CAD build for the part. Positions are in the model's coordinates, mm. Face numbers are marked on the shaded views. A direction names the side the tool comes from. Give positions to 0.01 mm unless a question says otherwise; leave off trailing zeros. Write each loop counter-clockwise with the first axis right and the second up, starting at its lowest first coordinate (ties: lowest second). Pieces come first, ordered by that corner, then holes. Notation, with made-up numbers: (21.5, 28.5) - (79.5, 28.5) arc R29 cw to (79.5, 66.5) - close; hole circle Ø8 at (-21, 41). An arc over 180 degrees is marked (long way). Put each result on its own line as item: value. Start each with the question number.
1. Drop flat-ended pins along their axis: pin 1 (1.5 mm diameter, centred on y = 454.5, z = 22, fed in from -X); pin 2 (11.5 mm diameter, centred on x = 22.5, z = 0, fed in from -Y); pin 3 (4 mm diameter, centred on y = 219.5, z = 0.5, fed in from +X); pin 4 (1 mm diameter, centred on x = 13, y = 62, fed in from -Z). Give the stop position or say it passes through.
2. Wall check: line 1 (Z direction, x = 0, y = 450.05); line 2 (X direction, y = 455.1, z = 0); line 3 (Z direction, x = 22.5, y = 451.1). Give the ranges that are in metal, low to high.
3. Tool access for the marked faces 4, 5 and 6: list every direction of +Z, -Z, +X, -X, +Y, -Y with a clear straight run to the whole face (end or side of a thin tool).
4. Mould opens along Y. For the marked faces 1, 2 and 3 say: +Y half, -Y half, draft (parallel to the pull), parting line (faces both ways), or undercut.
5. Cut at A-A on y = 79. List the corners of the cut face in (x, z), and give its area (3 significant figures).
from build123d import *

# Parameters (mm, degrees)
SKETCH1_W                     = 30
SKETCH1_H                     = 30
BOSS_EXTRUDE1_DEPTH           = 458
SKETCH2_W                     = 15
SKETCH2_H                     = 30
SKETCH2_W_2                   = 30
SKETCH2_H_2                   = 15
BOSS_EXTRUDE2_DEPTH           = 10
CBORE_FOR_M5_SHCS1_AT_2_COUNT = 2
CBORE_FOR_M5_SHCS1_AT_2_PITCH = 45
CBORE_FOR_M5_SHCS1_AT_3_COUNT = 2
CBORE_FOR_M5_SHCS1_AT_3_PITCH = 31.819805153
CBORE_FOR_M5_SHCS1_AT_4_COUNT = 2
CBORE_FOR_M5_SHCS1_AT_4_PITCH = 31.819805153
FILLET1_R                     = 5
FILLET1_OF_MIRROR1_R          = 5


with BuildPart() as part:
    # Sketch1 → Boss-Extrude1 (new body)
    with BuildSketch(Plane(origin=(0, 0, 0), x_dir=(1, 0, 0), z_dir=(0, 1, 0))):
        Rectangle(SKETCH1_W, SKETCH1_H)
    extrude(amount=BOSS_EXTRUDE1_DEPTH)

    # Sketch2 → Boss-Extrude2 (add)
    with BuildSketch(Plane(origin=(0, 0, 0), x_dir=(1, 0, 0), z_dir=(0, 1, 0))):
        with Locations((22.5, 0)):
            Rectangle(SKETCH2_W, SKETCH2_H)
        with Locations((0, -22.5)):
            Rectangle(SKETCH2_W_2, SKETCH2_H_2)
        with Locations((0, 22.5)):
            Rectangle(SKETCH2_W_2, SKETCH2_H_2)
        with Locations((-22.5, 0)):
            Rectangle(SKETCH2_W, SKETCH2_H)
    boss_extrude2 = extrude(amount=BOSS_EXTRUDE2_DEPTH)

    # Sketch4 → CBORE for M5 SHCS1 (revolve, cut)
    with BuildSketch(Plane(origin=(-22.5, 10, 0), x_dir=(0, 0, 1), z_dir=(1, 0, 0))):
        Polygon((0, 0), (0, 10), (2.75, 10), (2.75, 5), (5, 5), (5, 0.025), (5.025, 0), align=None)
    cbore_for_m5_shcs1 = revolve(axis=Axis((-22.5, 16.35, 0), (0, -1, 0)), mode=Mode.SUBTRACT)

    # CBORE for M5 SHCS1 at 2: CBORE for M5 SHCS1 ×2
    with Locations(*[(i * CBORE_FOR_M5_SHCS1_AT_2_PITCH, 0, 0) for i in range(1, CBORE_FOR_M5_SHCS1_AT_2_COUNT)]):
        add(cbore_for_m5_shcs1, mode=Mode.SUBTRACT)

    # CBORE for M5 SHCS1 at 3: CBORE for M5 SHCS1 ×2
    with Locations(*[Vector(0.7071067811865476, 0, -0.7071067811865476) * (i * CBORE_FOR_M5_SHCS1_AT_3_PITCH) for i in range(1, CBORE_FOR_M5_SHCS1_AT_3_COUNT)]):
        add(cbore_for_m5_shcs1, mode=Mode.SUBTRACT)

    # CBORE for M5 SHCS1 at 4: CBORE for M5 SHCS1 ×2
    with Locations(*[Vector(0.7071067811865476, 0, 0.7071067811865476) * (i * CBORE_FOR_M5_SHCS1_AT_4_PITCH) for i in range(1, CBORE_FOR_M5_SHCS1_AT_4_COUNT)]):
        add(cbore_for_m5_shcs1, mode=Mode.SUBTRACT)

    # Fillet1
    # the kernel refuses this fillet: 5 mm, written as the material it adds along each edge
    with BuildSketch(Plane(origin=(15, 0, 15), x_dir=(0, 0, 1), z_dir=(0, 1, 0)), Plane(origin=(15, 0, -15), x_dir=(1, 0, 0), z_dir=(0, 1, 0))) as fillet1_piece_1:
        with BuildLine():
            CenterArc((FILLET1_R, FILLET1_R), FILLET1_R, 180, 90)
            Line((0, FILLET1_R), (0, 0))
            Line((0, 0), (FILLET1_R, 0))
        make_face()
    extrude(amount=10)
    with BuildSketch(Plane(origin=(-15, 0, 15), x_dir=(0, 0, 1), z_dir=(0, 1, 0)), Plane(origin=(-15, 0, -15), x_dir=(-1, 0, 0), z_dir=(0, 1, 0))) as fillet1_piece_2:
        with BuildLine():
            CenterArc((FILLET1_R, -FILLET1_R), FILLET1_R, 90, 90)
            Line((0, -FILLET1_R), (0, 0))
            Line((0, 0), (FILLET1_R, 0))
        make_face()
    extrude(amount=10)
    # the kernel refuses this fillet: 5 mm, written as the material it takes off along each edge
    with BuildSketch(Plane(origin=(30, -12.5, 15), x_dir=(-1, 0, 0), z_dir=(0, 1, 0)), Plane(origin=(30, -12.5, -15), x_dir=(0, 0, 1), z_dir=(0, 1, 0)), Plane(origin=(-15, -12.5, 30), x_dir=(0, 0, -1), z_dir=(0, 1, 0)), Plane(origin=(15, -12.5, 30), x_dir=(-1, 0, 0), z_dir=(0, 1, 0)), Plane(origin=(-30, -12.5, -15), x_dir=(1, 0, 0), z_dir=(0, 1, 0))) as fillet1_2_piece_1:
        with BuildLine():
            CenterArc((FILLET1_R, -FILLET1_R), FILLET1_R, 90, 90)
            Line((0, -FILLET1_R), (0, 0))
            Line((0, 0), (FILLET1_R, 0))
        make_face()
    extrude(amount=35, mode=Mode.SUBTRACT)
    with BuildSketch(Plane(origin=(15, -12.5, -30), x_dir=(-1, 0, 0), z_dir=(0, 1, 0)), Plane(origin=(-15, -12.5, -30), x_dir=(0, 0, 1), z_dir=(0, 1, 0)), Plane(origin=(-30, -12.5, 15), x_dir=(1, 0, 0), z_dir=(0, 1, 0))) as fillet1_2_piece_2:
        with BuildLine():
            CenterArc((FILLET1_R, FILLET1_R), FILLET1_R, 180, 90)
            Line((0, FILLET1_R), (0, 0))
            Line((0, 0), (FILLET1_R, 0))
        make_face()
    extrude(amount=35, mode=Mode.SUBTRACT)

    # Mirror1: Boss-Extrude2, CBORE for M5 SHCS1 across plane
    add(boss_extrude2.mirror(Plane.ZX.offset(229)))
    add(cbore_for_m5_shcs1.mirror(Plane.ZX.offset(229)), mode=Mode.SUBTRACT)

    # Mirror1 copy 1 sketch → Mirror1 copy 1 (revolve, cut)
    with BuildSketch(Plane(origin=(22.5, 448, 0), x_dir=(0, 0, 1), z_dir=(1, 0, 0))):
        Polygon((0, 0), (0, -10), (2.75, -10), (2.75, -5), (5, -5), (5, -0.025), (5.025, 0), align=None)
    revolve(axis=Axis((22.5, 441.65, 0), (0, -1, 0)), mode=Mode.SUBTRACT)

    # Mirror1 copy 2 sketch → Mirror1 copy 2 (revolve, cut)
    with BuildSketch(Plane(origin=(0, 448, -22.5), x_dir=(0, 0, 1), z_dir=(1, 0, 0))):
        Polygon((0, 0), (0, -10), (2.75, -10), (2.75, -5), (5, -5), (5, -0.025), (5.025, 0), align=None)
    revolve(axis=Axis((0, 441.65, -22.5), (0, -1, 0)), mode=Mode.SUBTRACT)

    # Mirror1 copy 3 sketch → Mirror1 copy 3 (revolve, cut)
    with BuildSketch(Plane(origin=(0, 448, 22.5), x_dir=(0, 0, 1), z_dir=(1, 0, 0))):
        Polygon((0, 0), (0, -10), (2.75, -10), (2.75, -5), (5, -5), (5, -0.025), (5.025, 0), align=None)
    revolve(axis=Axis((0, 441.65, 22.5), (0, -1, 0)), mode=Mode.SUBTRACT)

    # Fillet1 of Mirror1
    # the kernel refuses this fillet: 5 mm, written as the material it adds along each edge
    with BuildSketch(Plane(origin=(15, 448, 15), x_dir=(0, 0, 1), z_dir=(0, 1, 0)), Plane(origin=(-15, 448, 15), x_dir=(-1, 0, 0), z_dir=(0, 1, 0))) as fillet1_of_mirror1_piece_1:
        with BuildLine():
            CenterArc((FILLET1_OF_MIRROR1_R, FILLET1_OF_MIRROR1_R), FILLET1_OF_MIRROR1_R, 180, 90)
            Line((0, FILLET1_OF_MIRROR1_R), (0, 0))
            Line((0, 0), (FILLET1_OF_MIRROR1_R, 0))
        make_face()
    extrude(amount=10)
    with BuildSketch(Plane(origin=(15, 448, -15), x_dir=(0, 0, -1), z_dir=(0, 1, 0)), Plane(origin=(-15, 448, -15), x_dir=(-1, 0, 0), z_dir=(0, 1, 0))) as fillet1_of_mirror1_piece_2:
        with BuildLine():
            CenterArc((FILLET1_OF_MIRROR1_R, -FILLET1_OF_MIRROR1_R), FILLET1_OF_MIRROR1_R, 90, 90)
            Line((0, -FILLET1_OF_MIRROR1_R), (0, 0))
            Line((0, 0), (FILLET1_OF_MIRROR1_R, 0))
        make_face()
    extrude(amount=10)
    # the kernel refuses this fillet: 5 mm, written as the material it takes off along each edge
    with BuildSketch(Plane(origin=(30, 470.5, 15), x_dir=(-1, 0, 0), z_dir=(0, -1, 0)), Plane(origin=(30, 470.5, -15), x_dir=(0, 0, 1), z_dir=(0, -1, 0)), Plane(origin=(-15, 470.5, 30), x_dir=(0, 0, -1), z_dir=(0, -1, 0)), Plane(origin=(15, 470.5, 30), x_dir=(-1, 0, 0), z_dir=(0, -1, 0)), Plane(origin=(-15, 470.5, -30), x_dir=(1, 0, 0), z_dir=(0, -1, 0)), Plane(origin=(-30, 470.5, -15), x_dir=(1, 0, 0), z_dir=(0, -1, 0))) as fillet1_of_mirror1_2_piece_1:
        with BuildLine():
            CenterArc((FILLET1_OF_MIRROR1_R, FILLET1_OF_MIRROR1_R), FILLET1_OF_MIRROR1_R, 180, 90)
            Line((0, FILLET1_OF_MIRROR1_R), (0, 0))
            Line((0, 0), (FILLET1_OF_MIRROR1_R, 0))
        make_face()
    extrude(amount=35, mode=Mode.SUBTRACT)
    with BuildSketch(Plane(origin=(15, 470.5, -30), x_dir=(-1, 0, 0), z_dir=(0, -1, 0)), Plane(origin=(-30, 470.5, 15), x_dir=(1, 0, 0), z_dir=(0, -1, 0))) as fillet1_of_mirror1_2_piece_2:
        with BuildLine():
            CenterArc((FILLET1_OF_MIRROR1_R, -FILLET1_OF_MIRROR1_R), FILLET1_OF_MIRROR1_R, 90, 90)
            Line((0, -FILLET1_OF_MIRROR1_R), (0, 0))
            Line((0, 0), (FILLET1_OF_MIRROR1_R, 0))
        make_face()
    extrude(amount=35, mode=Mode.SUBTRACT)


solid = part.part
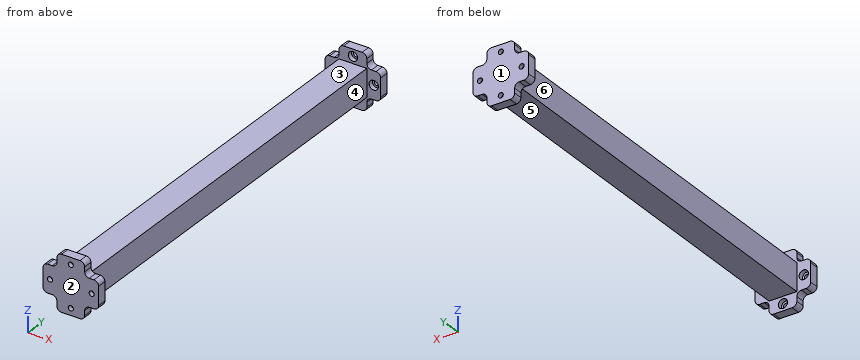
Report:
1. pin 1: stops at x = -15
1. pin 2: stops at y = 0
1. pin 3: stops at x = 15
1. pin 4: stops at z = -15
2. line 1: z = -30 to -27.5, -17.5 to 17.5, 27.5 to 30
2. line 2: x = -30 to -25.25, -19.75 to 19.75, 25.25 to 30
2. line 3: z = -15 to -5, 5 to 15
3. face 4: +Z, -Z, +X
3. face 5: -Z, +X, -X
3. face 6: +Z, -Z, -X
4. face 1: +Y half
4. face 2: -Y half
4. face 3: undercut
5. outline: (-15, -15) - (15, -15) - (15, 15) - (-15, 15) - close
5. area: 900 mm²
